The listing builds one solid part. Answer for the finished solid, in the listing's coordinates (mm). A direction names the side the tool comes from. Coordinates: 2 decimals unless noted, no trailing zeros. Loops run counter-clockwise (first coordinate to the right, second up) from the corner with the lowest first, then second, coordinate; pieces in that order, holes last. Notation, with made-up numbers: (-22, -10) - (25, -10) arc R20 ccw to (25, 11) - close; hole circle Ø10 at (-40, 62.5). An arc over 180 degrees is marked (long way). Return JSON: item names as keys, results as strings. Group by question number.
1. Each of these flat-tipped pins is pushed along its axis until it touches: P1, Ø2, axis at x = -13.5, y = -31.5, coming from the +Z side; P2, Ø1, axis at x = -20, y = -25, coming from the +Z side; P3, Ø12, axis at y = 39, z = -12, coming from the +X side; P4, Ø7, axis at x = -12, z = 22, coming from the +Y side. Where does it stop, or does it pass through?
2. Section B-B (y = 37.5) is taken. Write down the section's boundary in (x, z), and give its area (3 significant figures).
3. Which of the six approach directions +Z, -Z, +X, -X, +Y, -Y give full straight-line access (tool end or side, diameter ignored) to faces 1 (the face through (0, -32.017, 22)), 2 (the face through (0, 49.934, -19))?
4. Section C-C (z = 7) is taken. Write down the section's boundary in (x, y), and give its area (3 significant figures).
5. The mould has two halves that part along Z. Classify faces 3 (the face through (0, -35, 19.05)), 4 (the face through (30.939, -1, -19)), 5 (the face through (0, -38.367, 9)), 6 (the face through (0, -41, 25.4)): pulls with the +Z half, pulls with the -Z half, needs draft (parallel to the pull), parting line crosses it, or undercut.
6. Section A-A (x = -9) is taken. Write down the section's boundary in (y, z).
7. Find the intervals of material crossed by line 1 along Z through (x, y) = (-17, -33); line 2 along X through (y, z) = (-23.5, -1.5); line 3 along Z through (x, y) = (12, 43), in increasing order.
```python
from build123d import *

# Parameters (mm, degrees)
F1_W     = 61.967276
F1_H     = 11.567712
F2_DEPTH = 25.4
F0_W     = 61.878238
F0_H     = 99.868604
F3_DEPTH = 38.1
F4_W     = 61.967276
F4_H     = 6.35
F5_DEPTH = 6.35


with BuildPart() as f2:
    # F1 (on Top) → F2 (new body)
    with BuildSketch(Plane.XY):
        with Locations((0.029806, -44.150446)):
            Rectangle(F1_W, F1_H)
    extrude(amount=F2_DEPTH)

    # F0 (on Top) → F3 (join)
    with BuildSketch(Plane.XY):
        Rectangle(F0_W, F0_H)
    extrude(amount=-F3_DEPTH)

    # F4 (on face) → F5 (join)
    with BuildSketch(Plane(origin=(0, -38.36659, 0), x_dir=(-1, 0, 0), z_dir=(0, 1, 0))):
        with Locations((-0.029806, 22.225)):
            Rectangle(F4_W, F4_H)
    extrude(amount=F5_DEPTH)


solid = f2.part
```
The answers:
{
 "1": {"P1": "stops at z = 25.4", "P2": "stops at z = 0", "P3": "stops at x = 30.94", "P4": "stops at y = -32.02"},
 "2": {"outline": "(-30.94, -38.1) - (30.94, -38.1) - (30.94, 0) - (-30.94, 0) - close", "area": "2,360 mm2"},
 "3": {"face 1": "+Z, +X, -X, +Y", "face 2": "+Z, -Z, +X, -X, +Y"},
 "4": {"outline": "(-30.95, -49.93) - (31.01, -49.93) - (31.01, -38.37) - (-30.95, -38.37) - close", "area": "717 mm2"},
 "5": {"face 3": "undercut", "face 4": "needs draft", "face 5": "undercut", "face 6": "pulls with the +Z half"},
 "6": {"outline": "(-49.93, -38.1) - (49.93, -38.1) - (49.93, 0) - (-38.37, 0) - (-38.37, 19.05) - (-32.02, 19.05) - (-32.02, 25.4) - (-49.93, 25.4) - close"},
 "7": {"line 1": "z = -38.1 to 0, 19.05 to 25.4", "line 2": "x = -30.94 to 30.94", "line 3": "z = -38.1 to 0"}
}
